from build123d import *

# Parameters (mm, degrees)
SKETCH1_R           = 1
BOSS_EXTRUDE1_DEPTH = 5
BOSS_EXTRUDE2_DEPTH = 5
SKETCH3_R           = 1
CUT_EXTRUDE1_DEPTH  = 3


with BuildPart() as part:
    # Sketch1 → Boss-Extrude1 (new body)
    with BuildSketch(Plane(origin=(0, 0, 0), x_dir=(1, 0, 0), z_dir=(0, 1, 0))):
        with Locations(Location((0, 0, 0), (0, 0, 270))):
            Circle(SKETCH1_R)
    extrude(amount=BOSS_EXTRUDE1_DEPTH)

    # Sketch2 → Boss-Extrude2 (add)
    with BuildSketch(Plane(origin=(0, 0, 0), x_dir=(1, 0, 0), z_dir=(0, 1, 0))):
        Polygon((2.309401077, 0), (1.154700538, 2), (-1.154700538, 2), (-2.309401077, 0), (-1.154700538, -2), (1.154700538, -2), align=None)
    extrude(amount=-BOSS_EXTRUDE2_DEPTH)

    # Sketch3 → Cut-Extrude1 (cut)
    with BuildSketch(Plane.XZ.offset(5)):
        with Locations(Location((0, 0, 0), (0, 0, 90))):
            Circle(SKETCH3_R)
    extrude(amount=-CUT_EXTRUDE1_DEPTH, mode=Mode.SUBTRACT)


solid = part.part
Can you work these out from the model? Positions are in its coordinate system, mm. A direction names the side the tool comes from. Round coordinates to 2 decimals unless told otherwise and drop trailing zeros. Loops run counter-clockwise (first coordinate to the right, second up) from the corner with the lowest first, then second, coordinate; pieces in that order, holes last. Notation, with made-up numbers: (77, 59) - (100, 59) arc R14 ccw to (100, 76) - close; hole circle Ø5 at (-18, 13.5). An arc over 180 degrees is marked (long way). Answer in a Markdown table with one row per item. Add a question column.
Q1. I want a section at B-B on z = -0.5. List the corners of the cut face in (x, y) for me, and give its area (3 significant figures).
Q2. I want a section at C-C on y = 3.25. List the corners of the cut face in (x, z) for me, and give its area (3 significant figures).
Q3. Which directions (+Z, -Z, +X, -X, +Y, -Y) give clear straight access to the entire face, cutting with the end or side of a thin tool? Please do faces 1 (the flat face through (-1, 0, -1)), 2 (the flat face through (-1, -5, -1)).
Q4. We'd pull the mould along Z, two halves only. Please class faces 3 (the flat face through (0, -2, -2)), 4 (the cylindrical face through (-1, 2, 0)), 5 (the flat face through (0, -2, 0)), 6 (the cylindrical face through (1, -4, 0)): pulls with the +Z half, pulls with the -Z half, needs draft (parallel to the pull), parting line crosses it, or undercut.
Q5. For pin 1 Ø1.5 at (x, z) = (2, 1) entering from +Y; pin 2 Ø1 at (x, z) = (0, 0) entering from -Y; pin 3 Ø1.5 at (x, y) = (-1, 1.5) entering from +Z, each with a flat end and sliding along its axis, tell me the tip position at first contact or that it passes through.
Q6. I want a section at A-A on x = 0. List the corners of the cut face in (y, z) for me.
Q7. I need wall thicknesses on L1, parallel to Y at x = -0.55, z = -1.2; L2, parallel to Y at x = 0.2, z = 0.9; L3, parallel to Z at x = 0.3, y = -2.25. Which ranges of each line are inside material? Lowest first, please.
Q8. I want a section at D-D on x = 1.25. List the corners of the cut face in (y, z) for me, and give its area (3 significant figures).
A:
| question | item | result |
|---|---|---|
| 1 | outline | (-2.02, -5) - (-0.87, -5) - (-0.87, -2) - (0.87, -2) - (0.87, -5) - (2.02, -5) - (2.02, 0) - (0.87, 0) - (0.87, 5) - (-0.87, 5) - (-0.87, 0) - (-2.02, 0) - close |
| 1 | area | 23.7 mm^2 |
| 2 | outline | circle Ø2 at (0, 0) |
| 2 | area | 3.14 mm^2 |
| 3 | face 1 | +Y |
| 3 | face 2 | +Z, -Z, +X, -X, -Y |
| 4 | face 3 | pulls with the -Z half |
| 4 | face 4 | parting line crosses it |
| 4 | face 5 | undercut |
| 4 | face 6 | undercut |
| 5 | pin 1 | y = 0 |
| 5 | pin 2 | y = -2 |
| 5 | pin 3 | z = 0.97 |
| 6 | outline | (-5, -2) - (0, -2) - (0, -1) - (5, -1) - (5, 1) - (0, 1) - (0, 2) - (-5, 2) - (-5, 1) - (-2, 1) - (-2, -1) - (-5, -1) - close |
| 7 | L1 | -5 to 0 |
| 7 | L2 | -2 to 5 |
| 7 | L3 | -2 to -0.95, 0.95 to 2 |
| 8 | outline | (-5, -1.83) - (0, -1.83) - (0, 1.83) - (-5, 1.83) - close |
| 8 | area | 18.3 mm^2 |
